Geometry: final body of the model. Coordinates: model frame, mm. Face numbers are marked on the shaded views. A direction names the side the tool comes from. Give positions to 0.01 mm unless a question says otherwise; leave off trailing zeros. Write each loop counter-clockwise with the first axis right and the second up, starting at its lowest first coordinate (ties: lowest second). Pieces come first, ordered by that corner, then holes.
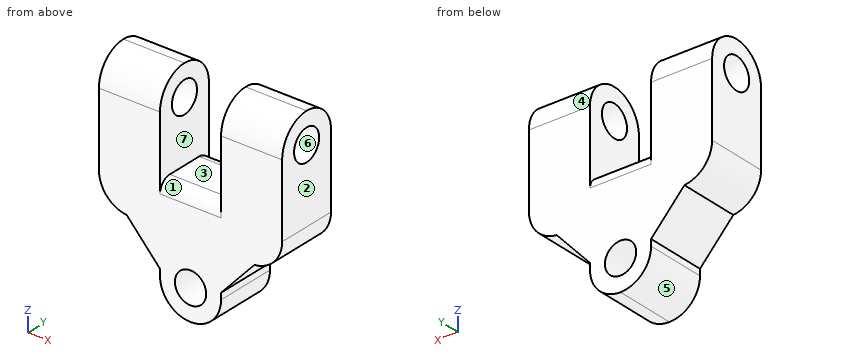
```python
from build123d import *

# Parameters (mm, degrees)
BOSS_EXTRUDE1_DEPTH = 3.175
FILLET1_R           = 3.175
CUT_EXTRUDE1_REACH  = 24.125
SKETCH2_R           = 1.627
SKETCH3_R           = 1.627
CUT_EXTRUDE2_DEPTH  = 6.35
SKETCH4_W           = 6.35
SKETCH4_H           = 6.35
CUT_EXTRUDE3_DEPTH  = 1.905
FILLET2_R           = 1.27
CHAMFER1_START      = -3.175
CHAMFER1_DEPTH      = 6.35


with BuildPart() as part:
    # Sketch1 → Boss-Extrude1 (new, symmetric)
    with BuildSketch(Plane(origin=(0, 0, 0), x_dir=(1, 0, 0), z_dir=(0, 1, 0))):
        Polygon((-3.175, 3.175), (-9.525, 3.175), (-9.525, -3.175), (-9.525, -10.795), (-3.175, -10.795), (-3.175, -3.175), (3.175, -3.175), (3.175, -10.795), (9.525, -10.795), (9.525, -3.175), (9.525, 3.175), (3.175, 3.175), (3.175, 10.795), (-3.175, 10.795), align=None)
    extrude(amount=BOSS_EXTRUDE1_DEPTH, both=True)

    # Fillet1
    fillet1_edges = [part.edges().sort_by_distance(p)[0] for p in [
        (3.175, 0, -10.795),
        (-3.175, 0, -10.795),
        (6.35, -3.175, 10.795),
        (6.35, 3.175, 10.795),
        (-6.35, -3.175, 10.795),
        (-6.35, 3.175, 10.795),
        (-9.525, 0, -3.175),
        (9.525, 0, -3.175),
    ]]
    fillet(fillet1_edges, radius=FILLET1_R - 0.0001)  # a hair under: the kernel refuses the full size

    # Cut-Extrude1: up to this face of the body (flat: up to its plane)
    cut_extrude1_end = Plane(part.part.faces().sort_by_distance((9.525, 0, 5.081615958))[0])
    # Sketch2 → Cut-Extrude1 (cut, up to the picked face)
    with BuildSketch(Plane.ZY.offset(9.525), mode=Mode.PRIVATE) as cut_extrude1_sk1:
        with Locations((7.62, 0)):
            Circle(SKETCH2_R)
    cut_extrude1_tool1 = split(extrude(cut_extrude1_sk1.sketch, amount=-CUT_EXTRUDE1_REACH, mode=Mode.PRIVATE), bisect_by=cut_extrude1_end, keep=Keep.BOTH, mode=Mode.PRIVATE)
    add(cut_extrude1_tool1.solids().sort_by(Axis((-9.525, 0, 7.62), (1, 0, 0)))[0], mode=Mode.SUBTRACT)

    # Sketch3 → Cut-Extrude2 (cut)
    with BuildSketch(Plane(origin=(0, 3.175, 0), x_dir=(1, 0, 0), z_dir=(0, 1, 0))):
        with Locations(Location((0, 7.62, 0), (0, 0, 270))):
            Circle(SKETCH3_R)
    extrude(amount=-CUT_EXTRUDE2_DEPTH, mode=Mode.SUBTRACT)

    # Sketch4 → Cut-Extrude3 (cut)
    with BuildSketch(Plane.XY.offset(3.175)):
        Rectangle(SKETCH4_W, SKETCH4_H)
    extrude(amount=-CUT_EXTRUDE3_DEPTH, mode=Mode.SUBTRACT)

    # Fillet2
    fillet2_edges = [part.edges().sort_by_distance(p)[0] for p in [
        (0, 3.175, 1.27),
        (0, -3.175, 1.27),
    ]]
    fillet(fillet2_edges, radius=FILLET2_R)

    # Chamfer1: read off the stored shape, not the designer's step
    # Chamfer1 outline → Chamfer1 (add)
    with BuildSketch(Plane(origin=(0, 0, 0), x_dir=(1, 0, 0), z_dir=(0, 1, 0)).offset(CHAMFER1_START)):
        with BuildLine():
            Line((6.638636364, 3.161852945), (3.175, 6.95607648))
            Line((3.175, 6.95607648), (3.175, 3.175))
            Line((3.175, 3.175), (6.35, 3.175))
            ThreePointArc((6.35, 3.175), (6.494467813, 3.171711533), (6.638636364, 3.161852945))
        make_face()
        with BuildLine():
            Line((-3.175, 6.95607648), (-6.638636364, 3.161852945))
            ThreePointArc((-6.638636364, 3.161852945), (-6.494467813, 3.171711533), (-6.35, 3.175))
            Line((-6.35, 3.175), (-3.175, 3.175))
            Line((-3.175, 3.175), (-3.175, 6.95607648))
        make_face()
    extrude(amount=CHAMFER1_DEPTH)


solid = part.part
```
Item 1: Section B-B, the plane x = 1.25. Return the cut outline in (y, z) (3 decimals).
Found:
outline: (-3.175, -10.539) - (3.175, -10.539) - (3.175, -8.661) - (-3.175, -8.661) - close; (-3.175, -6.579) - (3.175, -6.579) - (3.175, 0) arc R1.27 ccw to (1.905, 1.27) - (-1.905, 1.27) arc R1.27 ccw to (-3.175, 0) - close
Item 2: Pull-direction query (Z, two-part tool) for the marked faces 4, 5, 6 and 7; classes: +Z half, -Z half, draft (parallel to the pull), parting line (faces both ways), or undercut.
Found:
face 4: +Z half
face 5: -Z half
face 6: undercut
face 7: draft
Item 3: Line query: L1, parallel to X at y = 2, z = 8 (3 decimals); L2, parallel to X at y = -1, z = -7.62 (3 decimals). Output: solid intervals per line, ascending.
Found:
L1: x = -9.525 to -3.175, 3.175 to 9.525
L2: x = -3.175 to -1.627, 1.627 to 3.175
Item 4: Section A-A, the plane y = 1. State how many separate pieces and enclosed holes the cut face has, plus the area to 3 significant figures.
Found:
separate pieces: 3
enclosed holes: 1
area: 215 mm2
Item 5: Reachability of the marked faces 1, 2 and 3 from +Z, -Z, +X, -X, +Y, -Y: full face, straight path, thin tool, end or side. Return the list, or none.
Found:
face 1: +Z, -Y
face 2: +Z, -Z, +X, +Y, -Y
face 3: +Z, +Y, -Y
Item 6: Pin query (flat end, axial travel): pin 1 Ø0.7 at (y, z) = (-0.5, -7.5) entering from +X (3 decimals); pin 2 Ø0.7 at (y, z) = (0.5, -7.5) entering from -X (3 decimals); pin 3 Ø1.5 at (x, y) = (-6.5, -1) entering from -Z. Return the tip coordinate at first contact, or that it passes through.
Found:
pin 1: stops at x = 3.175
pin 2: stops at x = -3.175
pin 3: stops at z = -4.14
